Geometry check sheet. Reference: the model listing, model coordinates, mm. Coordinates: 2 decimals unless noted, no trailing zeros. Write each loop counter-clockwise with the first axis right and the second up, starting at its lowest first coordinate (ties: lowest second). Pieces come first, ordered by that corner, then holes. Notation, with made-up numbers: (89.5, 17) -> (143.5, 17) arc R16 ccw to (143.5, 24) -> close; hole circle Ø4 at (8, 26). An arc over 180 degrees is marked (long way). Answer in a Markdown table with one row per item. Add a question column.
Q1. Thickness scan on line 1 (Z direction, x = 17.5, y = 2.45); line 2 (X direction, y = 1, z = -17.5); line 3 (Z direction, x = 15.5, y = 3.4). Record the ranges inside material, lowest first.
Q2. Section check C-C, the plane z = -17.5. Record the boundary of the cut face in (x, y), and give its area (3 significant figures).
Q3. Section check D-D, the plane z = -32. Record the boundary of the cut face in (x, y).
Q4. Release check for a two-part mould opening along Z. For faces 1 (the face through (15, 2, -17.6)), 2 (the face through (17, 2, 0)), 3 (the face through (17, 0, -14)), 4 (the face through (32.4, 2, -32.3)) record: pulls with the +Z half, pulls with the -Z half, needs draft (parallel to the pull), parting line crosses it, or undercut.
Q5. Section check A-A, the plane x = 17.5. Record the boundary of the cut face in (y, z).
Q6. Section check B-B, the plane y = 1.15. Record the boundary of the cut face in (x, z).
```python
from build123d import *

# Parameters (mm, degrees)
CROQUIS1_W              = 35
CROQUIS1_H              = 35
SALIENTE_EXTRUIR1_DEPTH = 4
CROQUIS2_OUTSIDE_W      = 46.932
CROQUIS2_OUTSIDE_H      = 46.932
CORTAR_EXTRUIR2_DEPTH   = 18
CROQUIS3_R              = 2.5
CORTAR_EXTRUIR3_DEPTH   = 5


with BuildPart() as part:
    # Croquis1 → Saliente-Extruir1 (new body)
    with BuildSketch(Plane(origin=(0, 0, 0), x_dir=(1, 0, 0), z_dir=(0, 1, 0))):
        with Locations((17.5, 17.5)):
            Rectangle(CROQUIS1_W, CROQUIS1_H)
    extrude(amount=SALIENTE_EXTRUIR1_DEPTH)

    # Croquis2 outside → Cortar-Extruir2 (cut)
    with BuildSketch(Plane(origin=(0, 4, 0), x_dir=(1, 0, 0), z_dir=(0, 1, 0))):
        with Locations((17.5, 17.5)):
            Rectangle(CROQUIS2_OUTSIDE_W, CROQUIS2_OUTSIDE_H)
        Polygon((5.30151519, 35), (0, 29.69848481), (0, 5.30151519), (5.30151519, 0), (29.69848481, 0), (35, 5.30151519), (35, 29.69848481), (29.69848481, 35), align=None, mode=Mode.SUBTRACT)
    extrude(amount=-CORTAR_EXTRUIR2_DEPTH, mode=Mode.SUBTRACT)

    # Croquis3 → Cortar-Extruir3 (cut, through all)
    with BuildSketch(Plane(origin=(0, 4, 0), x_dir=(1, 0, 0), z_dir=(0, 1, 0))):
        with Locations((17.5, 17.5)):
            Circle(CROQUIS3_R)
    extrude(amount=-CORTAR_EXTRUIR3_DEPTH, mode=Mode.SUBTRACT)


solid = part.part
```
Calculated:
| question | item | result |
|---|---|---|
| 1 | line 1 | z = -35 to -20, -15 to 0 |
| 1 | line 2 | x = 0 to 15, 20 to 35 |
| 1 | line 3 | z = -35 to -19, -16 to 0 |
| 2 | outline | (0, 0) -> (15, 0) -> (15, 4) -> (0, 4) -> close; (20, 0) -> (35, 0) -> (35, 4) -> (20, 4) -> close |
| 2 | area | 120 mm² |
| 3 | outline | (2.3, 0) -> (32.7, 0) -> (32.7, 4) -> (2.3, 4) -> close |
| 4 | face 1 | undercut |
| 4 | face 2 | pulls with the +Z half |
| 4 | face 3 | needs draft |
| 4 | face 4 | pulls with the -Z half |
| 5 | outline | (0, -35) -> (4, -35) -> (4, -20) -> (0, -20) -> close; (0, -15) -> (4, -15) -> (4, 0) -> (0, 0) -> close |
| 6 | outline | (0, -29.7) -> (5.3, -35) -> (29.7, -35) -> (35, -29.7) -> (35, -5.3) -> (29.7, 0) -> (5.3, 0) -> (0, -5.3) -> close; hole circle Ø5 at (17.5, -17.5) |
